Work out the finished part from the listing and answer in its coordinate system (mm). A direction names the side the tool comes from. Give positions to 0.01 mm unless a question says otherwise; leave off trailing zeros. Loops run counter-clockwise (first coordinate to the right, second up) from the corner with the lowest first, then second, coordinate; pieces in that order, holes last.
```python
from build123d import *

# Parameters (mm, degrees)
SKETCH1_R           = 1.5
SKETCH1_R_2         = 4
BOSS_EXTRUDE1_DEPTH = 15
CUT_EXTRUDE1_START  = -11
CUT_EXTRUDE1_DEPTH  = 7


with BuildPart() as part:
    # Sketch1 → Boss-Extrude1 (new body)
    with BuildSketch(Plane.XY):
        with BuildLine():
            Line((-32, 0), (32, 0))
            ThreePointArc((32, 0), (40, 8), (32, 16))
            Line((32, 16), (18.027756377, 16))
            ThreePointArc((18.027756377, 16), (10.00991912, 17.09127665), (2.575393768, 20.285714286))
            ThreePointArc((2.575393768, 20.285714286), (0, 21), (-2.575393768, 20.285714286))
            ThreePointArc((-2.575393768, 20.285714286), (-10.00991912, 17.09127665), (-18.027756377, 16))
            Line((-18.027756377, 16), (-32, 16))
            ThreePointArc((-32, 16), (-40, 8), (-32, 0))
        make_face()
        with Locations((0, 18)):
            Circle(SKETCH1_R, mode=Mode.SUBTRACT)
        with Locations((-32, 8)):
            Circle(SKETCH1_R_2, mode=Mode.SUBTRACT)
        with Locations((32, 8)):
            Circle(SKETCH1_R_2, mode=Mode.SUBTRACT)
    extrude(amount=BOSS_EXTRUDE1_DEPTH)

    # Sketch2 → Cut-Extrude1 (cut)
    with BuildSketch(Plane.XY.offset(15).offset(CUT_EXTRUDE1_START)):
        with BuildLine():
            Line((-18.027756377, 16), (-15, 16))
            ThreePointArc((-15, 16), (-8.67544468, 14.973665961), (-3, 12))
            ThreePointArc((-3, 12), (0, 11), (3, 12))
            ThreePointArc((3, 12), (8.67544468, 14.973665961), (15, 16))
            Line((15, 16), (18.027756377, 16))
            Line((18.027756377, 16), (18.027756377, 21))
            Line((18.027756377, 21), (-18.027756377, 21))
            Line((-18.027756377, 21), (-18.027756377, 16))
        make_face()
    extrude(amount=CUT_EXTRUDE1_DEPTH, mode=Mode.SUBTRACT)


solid = part.part
```
Q1. Determine the mould class of faces 3 (the face through (-1, 8, 0)), 4 (the face through (40, 8, 7)), 5 (the face through (0, 16, 11)) for opening direction Z: +Z half, -Z half, draft (parallel to the pull), parting line (faces both ways), or undercut.
Q2. Section C-C on z = 10 is taken. Give the vertices of the cut face in (x, y), plus the area to 3 significant figures.
Q3. Given pin 1 (4 mm diameter, centred on y = 5, z = 6, fed in from -X); pin 2 (5 mm diameter, centred on y = 5, z = 3.5, fed in from +X); pin 3 (6.5 mm diameter, centred on x = -32, y = 8, fed in from -Z); pin 4 (7.5 mm diameter, centred on x = 24.5, z = 5.5, fed in from +Y), each flat-ended and moving along its own axis, determine where each tip first touches the part or whether it passes through.
Q4. Section D-D on y = 18 is taken. Give the vertices of the cut face in (x, z).
Q5. Which of the six approach directions +Z, -Z, +X, -X, +Y, -Y give full straight-line access (tool end or side, diameter ignored) to faces 1 (the face through (8.59, 14.945, 7.451)), 2 (the face through (-9.9, 17.12, 1.97))?
Q6. Section B-B on y = 8 is taken. Give the vertices of the cut face in (x, z).
Q7. Consider line 1 along Y through (x, z) = (32, 4.5); line 2 along X through (y, z) = (7.25, 13); line 3 along Y through (x, z) = (0, 13.1). Determine where each line is inside the solid, lowest interval first.
Q8. Section A-A on x = 0 is taken. Give the vertices of the cut face in (y, z), plus the area to 3 significant figures.
Check result:
1. face 3: -Z half
1. face 4: draft
1. face 5: undercut
2. outline: (-32, 0) - (32, 0) arc R8 ccw to (32, 16) - (15, 16) arc R20 ccw to (3, 12) arc R5 cw to (-3, 12) arc R20 ccw to (-15, 16) - (-32, 16) arc R8 ccw to start; hole circle Ø8 at (-32, 8); hole circle Ø8 at (32, 8)
2. area: 1,070 mm2
3. pin 1: stops at x = -39.94
3. pin 2: stops at x = 39.98
3. pin 3: passes through
3. pin 4: stops at y = 16
4. outline: (-7.26, 0) - (-1.5, 0) - (-1.5, 4) - (-7.26, 4) - close; (-7.26, 11) - (-1.5, 11) - (-1.5, 15) - (-7.26, 15) - close; (1.5, 0) - (7.26, 0) - (7.26, 4) - (1.5, 4) - close; (1.5, 11) - (7.26, 11) - (7.26, 15) - (1.5, 15) - close
5. face 1: +Y
5. face 2: +Z, -Z, -X, +Y
6. outline: (-40, 0) - (-36, 0) - (-36, 15) - (-40, 15) - close; (-28, 0) - (28, 0) - (28, 15) - (-28, 15) - close; (36, 0) - (40, 0) - (40, 15) - (36, 15) - close
7. line 1: y = 0 to 4, 12 to 16
7. line 2: x = -39.96 to -35.93, -28.07 to 28.07, 35.93 to 39.96
7. line 3: y = 0 to 16.5, 19.5 to 21
8. outline: (0, 0) - (16.5, 0) - (16.5, 4) - (11, 4) - (11, 11) - (16.5, 11) - (16.5, 15) - (0, 15) - close; (19.5, 0) - (21, 0) - (21, 4) - (19.5, 4) - close; (19.5, 11) - (21, 11) - (21, 15) - (19.5, 15) - close
8. area: 221 mm2
